Geometry: final body of the model. Coordinates: model frame, mm. Face numbers are marked on the shaded views. A direction names the side the tool comes from. Give positions to 0.01 mm unless a question says otherwise; leave off trailing zeros. Write each loop counter-clockwise with the first axis right and the second up, starting at its lowest first coordinate (ties: lowest second). Pieces come first, ordered by that corner, then holes. Notation, with made-up numbers: M 42.5,66 L 47.5,66 A25 cw 47.5,88 Z; hole C -25.5,64.25 d9. An arc over 180 degrees is marked long. Answer as a JSON object with one key per item and string values.
from build123d import *

# Parameters (mm, degrees)
TYKKELSE_LEDDFESTER_OG_BREDDE_H_YDE_SELV_DEPTH = 13
SKETCH28_R                                     = 15.5
SKETCH28_R_2                                   = 10.5
HULL_TIL_L_RBEN_KARBONFIBERR_R_DEPTH           = 10
SKRUEHULL_LEDDFESTER_DEPTH                     = 167.325734629
SKRUEHULL_LEDDFESTER_DEPTH_BACK                = 167.325734629
SKETCH29_R                                     = 3
SKETCH33_W                                     = 5
SKETCH33_H                                     = 20
BREDDE_OG_AVSTAND_STEMPELENDE_DEPTH            = 60
CUT_EXTRUDE4_DEPTH                             = 148.147035308
SIDEM_NSTER_DEPTH                              = 9.088039
SIDEM_NSTER_2_DEPTH                            = 9.088039
UTVIDET_START                                  = -60
SKETCH44_R                                     = 10.5
UTVIDET_L_RBENHULL_INN_I_SELVE_KROPPEN_DEPTH   = 60
M_NSTER_TOPP_DEPTH                             = 10
STEMPELENDE_AV_ST_RSTE_SYLINDER_DEPTH          = 145.150962536
STEMPELENDE_AV_ST_RSTE_SYLINDER_DEPTH_BACK     = 145.150962536
ROD_ENDE_JUSTERE_LENGDEN_ALTS_FESTE_T_R        = 3
SKETCH39_W                                     = 5
SKETCH39_H                                     = 15
SYLINDERFESTE_SELVE_DEN_LILLE_SYLINDERE_DEPTH  = 25
ST_TTER_ST_RSTE_SYLINDER_1_DEPTH               = 5
ST_TTER_ST_RSTE_SYLINDER_2_DEPTH               = 5
SYLINDERFESTE_LITEN_SYLINDER_DEPTH             = 134.515916654
SYLINDERFESTE_LITEN_SYLINDER_DEPTH_BACK        = 134.515916654
SKETCH48_R                                     = 2.5
BOSS_EXTRUDE11_DEPTH                           = 5
BOSS_EXTRUDE12_DEPTH                           = 5
SKETCH51_R                                     = 10
TIL_ASSEMBLY_SLETT_F_R_PRINTING_DEPTH          = 170


with BuildPart() as part:
    # Sketch27 → Tykkelse leddfester og bredde/høyde selve modellen (new, symmetric)
    with BuildSketch(Plane.XY):
        Polygon((66, -50), (-66, -50), (-66, 100), (-60, 100), (-60, 70), (60, 70), (60, 100), (66, 100), align=None)
    extrude(amount=TYKKELSE_LEDDFESTER_OG_BREDDE_H_YDE_SELV_DEPTH, both=True)

    # Sketch28 → Hull til lårben/karbonfiberrør (add)
    with BuildSketch(Plane.XZ.offset(50)):
        with Locations(Location((0, 0, 0), (0, 0, 57.004114526))):
            Circle(SKETCH28_R)
        with Locations(Location((0, 0, 0), (0, 0, 270))):
            Circle(SKETCH28_R_2, mode=Mode.SUBTRACT)
    extrude(amount=HULL_TIL_L_RBEN_KARBONFIBERR_R_DEPTH)

    # Sketch29 → Skruehull leddfester (cut, two sides: drawn at the far end of the back side and taken through both)
    with BuildSketch(Plane(origin=(66, 0, 0), x_dir=(0, 0, -1), z_dir=(1, 0, 0)).offset(-SKRUEHULL_LEDDFESTER_DEPTH_BACK)):
        with Locations((0, 86.5)):
            Circle(SKETCH29_R)
        with BuildLine():
            Line((-13, 86.5), (-13, 71.5))
            Line((-13, 71.5), (-14, 71.5))
            Line((-14, 71.5), (-14, 101))
            Line((-14, 101), (0, 101))
            Line((0, 101), (14, 101))
            Line((14, 101), (14, 71.5))
            Line((14, 71.5), (13, 71.5))
            Line((13, 71.5), (13, 86.5))
            ThreePointArc((13, 86.5), (0, 99.5), (-13, 86.5))
        make_face()
    extrude(amount=SKRUEHULL_LEDDFESTER_DEPTH + SKRUEHULL_LEDDFESTER_DEPTH_BACK, mode=Mode.SUBTRACT)

    # Sketch33 → Bredde og avstand stempelende (add)
    with BuildSketch(Plane(origin=(0, 0, -13), x_dir=(-1, 0, 0), z_dir=(0, 0, -1))):
        with Locations((-6, -40)):
            Rectangle(SKETCH33_W, SKETCH33_H)
        with Locations((6, -40)):
            Rectangle(SKETCH33_W, SKETCH33_H)
    extrude(amount=BREDDE_OG_AVSTAND_STEMPELENDE_DEPTH)

    # Fasong (mønster på selve kroppen) → Cut-Extrude4 (cut, through all)
    with BuildSketch(Plane.XY.offset(13)):
        Polygon((-66, 60), (-15.5, -50), (-66, -50), align=None)
        Polygon((15.5, -50), (66, -50), (66, 60), align=None)
        Polygon((-56, 60), (-15.5, -28.217821782), (-15.5, 60), align=None)
        Polygon((56, 60), (15.5, 60), (15.5, -28.217821782), align=None)
    extrude(amount=-CUT_EXTRUDE4_DEPTH, mode=Mode.SUBTRACT)

    # Sketch40 → Sidemønster (cut)
    with BuildSketch(Plane(origin=(-31.760550161, -14.580979847, 0), x_dir=(0, 0, 1), z_dir=(-0.9088038689830882, -0.41722359439678147, 0))):
        Polygon((-8, 75.564989369), (8, 75.564989369), (8, 59.564989369), align=None)
        Polygon((-8, 68.493921557), (8, 52.493921557), (-8, 36.493921557), align=None)
        Polygon((8, 13.422853745), (-8, 29.422853745), (8, 45.422853745), align=None)
        Polygon((-8, 22.351785934), (8, 6.351785934), (-8, 6.351785934), align=None)
    extrude(amount=-SIDEM_NSTER_DEPTH, mode=Mode.SUBTRACT)

    # Sketch42 → Sidemønster 2 (cut)
    with BuildSketch(Plane(origin=(31.760550161, -14.580979847, 0), x_dir=(0, 0, -1), z_dir=(0.9088038689830882, -0.41722359439678147, 0))):
        Polygon((8, 75.564989369), (-8, 75.564989369), (-8, 59.564989369), align=None)
        Polygon((8, 68.493921557), (-8, 52.493921557), (8, 36.493921557), align=None)
        Polygon((-8, 45.422853745), (8, 29.422853745), (-8, 13.422853745), align=None)
        Polygon((8, 22.351785934), (-8, 6.351785934), (8, 6.351785934), align=None)
    extrude(amount=-SIDEM_NSTER_2_DEPTH, mode=Mode.SUBTRACT)

    # Sketch44 → Utvidet lårbenhull inn i selve kroppen (cut)
    with BuildSketch(Plane.XZ.offset(50).offset(UTVIDET_START)):
        with Locations(Location((0, 0, 0), (0, 0, 270))):
            Circle(SKETCH44_R)
    extrude(amount=UTVIDET_L_RBENHULL_INN_I_SELVE_KROPPEN_DEPTH, mode=Mode.SUBTRACT)

    # Sketch45 → Mønster topp (cut)
    with BuildSketch(Plane(origin=(0, 70, 0), x_dir=(1, 0, 0), z_dir=(0, 1, 0))):
        Polygon((-39.928932188, 10.5), (-31.928932188, 2.5), (-23.928932188, 10.5), align=None)
        Polygon((-16.857864376, 10.5), (-8.857864376, 2.5), (-8.857864376, 10.5), align=None)
        Polygon((-55, 2.5), (-55, 10.5), (-47, 10.5), align=None)
        Polygon((-43.464466094, 10.5), (-51.464466094, 2.5), (-35.464466094, 2.5), align=None)
        Polygon((-20.393398282, 10.5), (-28.393398282, 2.5), (-12.393398282, 2.5), align=None)
        Polygon((-8.857864376, -2.5), (-8.857864376, -10.5), (-16.857864376, -10.5), align=None)
        Polygon((-20.393398282, -10.5), (-12.393398282, -2.5), (-28.393398282, -2.5), align=None)
        Polygon((-23.928932188, -10.5), (-31.928932188, -2.5), (-39.928932188, -10.5), align=None)
        Polygon((-43.464466094, -10.5), (-35.464466094, -2.5), (-51.464466094, -2.5), align=None)
        Polygon((-55, -10.5), (-47, -10.5), (-55, -2.5), align=None)
        Polygon((8.857864376, 2.5), (8.857864376, 10.5), (16.857864376, 10.5), align=None)
        Polygon((16.857864376, -10.5), (8.857864376, -2.5), (8.857864376, -10.5), align=None)
        Polygon((20.393398282, -10.5), (28.393398282, -2.5), (12.393398282, -2.5), align=None)
        Polygon((20.393398282, 10.5), (12.393398282, 2.5), (28.393398282, 2.5), align=None)
        Polygon((23.928932188, 10.5), (31.928932188, 2.5), (39.928932188, 10.5), align=None)
        Polygon((23.928932188, -10.5), (39.928932188, -10.5), (31.928932188, -2.5), align=None)
        Polygon((43.464466094, -10.5), (51.464466094, -2.5), (35.464466094, -2.5), align=None)
        Polygon((55, -2.5), (55, -10.5), (47, -10.5), align=None)
        Polygon((43.464466094, 10.5), (35.464466094, 2.5), (51.464466094, 2.5), align=None)
        Polygon((55, 10.5), (47, 10.5), (55, 2.5), align=None)
    extrude(amount=-M_NSTER_TOPP_DEPTH, mode=Mode.SUBTRACT)

    # Rod-ende, justere lengden (altså feste til største sylinder) → Stempelende av st_rste sylinder (cut, two sides: drawn at the far end of the back side and taken through both)
    with BuildSketch(Plane(origin=(8.5, 0, 0), x_dir=(0, 0, -1), z_dir=(1, 0, 0)).offset(-STEMPELENDE_AV_ST_RSTE_SYLINDER_DEPTH_BACK)):
        with Locations((33, -40)):
            Circle(ROD_ENDE_JUSTERE_LENGDEN_ALTS_FESTE_T_R)
        with BuildLine():
            Line((43, -51), (74, -51))
            Line((74, -51), (74, -29))
            Line((74, -29), (43, -29))
            Line((43, -29), (13, -29))
            Line((13, -29), (13, -31))
            Line((13, -31), (33, -31))
            ThreePointArc((33, -31), (42, -40), (33, -49))
            Line((33, -49), (13, -49))
            Line((13, -49), (13, -51))
            Line((13, -51), (43, -51))
        make_face()
    extrude(amount=STEMPELENDE_AV_ST_RSTE_SYLINDER_DEPTH + STEMPELENDE_AV_ST_RSTE_SYLINDER_DEPTH_BACK, mode=Mode.SUBTRACT)

    # Sketch39 → Sylinderfeste_ selve den lille sylindere (add)
    with BuildSketch(Plane.XY.offset(13)):
        with Locations((-10, -22.5)):
            Rectangle(SKETCH39_W, SKETCH39_H)
        with Locations((10, -22.5)):
            Rectangle(SKETCH39_W, SKETCH39_H)
    extrude(amount=SYLINDERFESTE_SELVE_DEN_LILLE_SYLINDERE_DEPTH)

    # Sketch46 → Støtter største sylinder 1 (add)
    with BuildSketch(Plane(origin=(8.5, 0, 0), x_dir=(0, 0, -1), z_dir=(1, 0, 0))):
        Polygon((13, -6), (13, -14.003905297), (26.596875763, -31), (33, -31), align=None)
    extrude(amount=-ST_TTER_ST_RSTE_SYLINDER_1_DEPTH)

    # Sketch47 → Støtter største sylinder 2 (add)
    with BuildSketch(Plane.ZY.offset(8.5)):
        Polygon((-33, -31), (-13, -6), (-13, -14.003905297), (-26.596875763, -31), align=None)
    extrude(amount=-ST_TTER_ST_RSTE_SYLINDER_2_DEPTH)

    # Sketch48 → Sylinderfeste, liten sylinder (cut, two sides: drawn at the far end of the back side and taken through both)
    with BuildSketch(Plane.ZY.offset(12.5).offset(-SYLINDERFESTE_LITEN_SYLINDER_DEPTH_BACK)):
        with Locations(Location((28, -22.5, 0), (0, 0, 270))):
            Circle(SKETCH48_R)
        with BuildLine():
            Line((28, -30), (13.179811187, -30))
            Line((13.179811187, -30), (13.179811187, -31))
            Line((13.179811187, -31), (39, -31))
            Line((39, -31), (39, -14))
            Line((39, -14), (13, -14))
            Line((13, -14), (13, -15))
            Line((13, -15), (28, -15))
            ThreePointArc((28, -15), (35.5, -22.5), (28, -30))
        make_face()
    extrude(amount=SYLINDERFESTE_LITEN_SYLINDER_DEPTH + SYLINDERFESTE_LITEN_SYLINDER_DEPTH_BACK, mode=Mode.SUBTRACT)

    # Sketch49 → Boss-Extrude11 (add)
    with BuildSketch(Plane.ZY.offset(12.5)):
        Polygon((28, -35), (13, -10), (13, -19.718253158), (22.169048105, -35), align=None)
    extrude(amount=-BOSS_EXTRUDE11_DEPTH)

    # Sketch50 → Boss-Extrude12 (add)
    with BuildSketch(Plane(origin=(12.5, 0, 0), x_dir=(0, 0, -1), z_dir=(1, 0, 0))):
        Polygon((-28, -35), (-22.169048105, -35), (-13, -19.718253158), (-13, -10), align=None)
    extrude(amount=-BOSS_EXTRUDE12_DEPTH)

    # Sketch51 → TIL ASSEMBLY - SLETT FØR PRINTING (add)
    with BuildSketch(Plane.XZ.offset(-10)):
        with Locations(Location((0, 0, 0), (0, 0, 270))):
            Circle(SKETCH51_R)
    extrude(amount=TIL_ASSEMBLY_SLETT_F_R_PRINTING_DEPTH)


solid = part.part
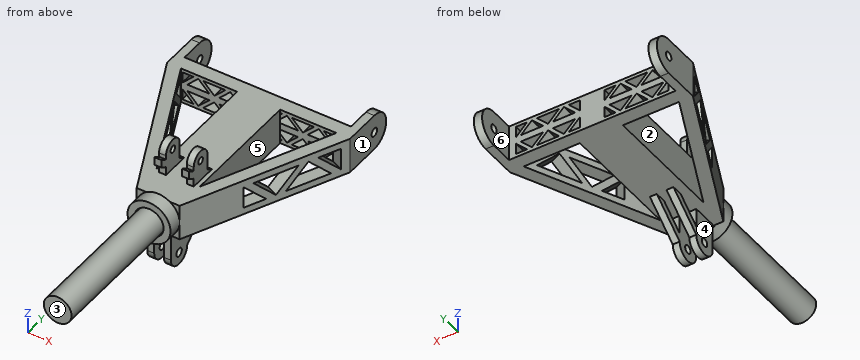
1) Set-up query: the marked faces 4, 5 and 6. Return all of +Z, -Z, +X, -X, +Y, -Y with unobstructed straight access to the full face (end or side cutting, diameter ignored); none if empty.
Geometry check:
{"face 4": "-Z, -X, +Y, -Y", "face 5": "+Z, -Z", "face 6": "+Z, -Z, +Y"}
2) Line query: line 1 (Z direction, x = 9, y = -22); line 2 (X direction, y = -35.5, z = 0); line 3 (Y direction, x = 7.35, z = -33). Output: solid intervals per line, ascending. Write a range as from..to.
Geometry check:
{"line 1": "z = -13..-5.41, -4.36..4.36, 5.41..25.55, 30.45..35.48", "line 2": "x = -22.16..-10.5, -10..10, 10.5..22.16", "line 3": "y = -49..-43, -37..-31"}
3) Cut plane B-B on y = -143. Return loops of the section in (x, z), and give its area (3 significant figures).
Geometry check:
{"outline": "C 0,0 d20", "area": "314 mm2"}
4) Pull-direction query (X, two-part tool) for the marked faces 1, 2 and 3; classes: pulls with the +X half, pulls with the -X half, needs draft (parallel to the pull), parting line crosses it, or undercut.
Geometry check:
{"face 1": "pulls with the +X half", "face 2": "undercut", "face 3": "needs draft"}
5) Contact query for flat-ended pins moving along their axis: P1, Ø3, axis at x = 0.5, z = 1, coming from the +Y side; P2, Ø5, axis at x = -39.5, y = 66, coming from the -Z side; P3, Ø5.5, axis at x = -10.5, z = 3.5, coming from the -Y side; P4, Ø5, axis at x = -9, y = 73.5, coming from the +Z side. Output: stop coordinate, or through.
Geometry check:
{"P1": "stops at y = 70", "P2": "stops at z = -13", "P3": "stops at y = -160", "P4": "passes through"}
6) Cut plane A-A on y = -40. Return loops of the section in (x, z).
Geometry check:
{"outline": "M -20.09,-13 L -8.5,-13 L -8.5,-30 L -3.5,-30 L -3.5,-13 L 3.5,-13 L 3.5,-30 L 8.5,-30 L 8.5,-13 L 20.09,-13 L 20.09,13 L -20.09,13 Z; C 0,0 d20; M -8.5,-42 L -3.5,-42 L -3.5,-36 L -8.5,-36 Z; M 3.5,-42 L 8.5,-42 L 8.5,-36 L 3.5,-36 Z; hole C 0,0 d21"}
